Source: CAD feature listing. Evaluate the final solid. Frame: model axes, mm. A direction names the side the tool comes from. Coordinates: 2 decimals unless noted, no trailing zeros. Order: outer loops, then holes, each group sorted by start corner. A loop starts at its lowest first (then second) coordinate and runs counter-clockwise, first axis right, second up. Notation, with made-up numbers: (27, 12.25) -> (63, 12.25) arc R13 cw to (63, 16.25) -> close; hole circle Ø5 at (23.5, 1). An arc over 180 degrees is marked (long way). Write each question's results on one line, items separated by ' | '. Start each with the question number.
Solid Edge part; units mm, degrees
sketch "Sketch1" plane through (0, 0, 0) normal (0, -1, 0) x (1, 0, 0)
  line L0 (21, -100) -> (21, 100)
  line L1 (21, 100) -> (-21, 100)
  line L2 (-21, 100) -> (-21, -100)
  line L3 (-21, -100) -> (21, -100)
extrude "Protrusion1" add sketch "Sketch1" along normal blind 10
sketch "Sketch2" plane through (0, 0, 0) normal (0, -1, 0) x (1, 0, 0)
  circle A0 centre (16, -56.5) radius 2
  circle A1 centre (-16, -56.5) radius 2
  circle A2 centre (-16, -90) radius 2
  circle A3 centre (16, -90) radius 2
extrude "ExtrudedProtrusion_2" add sketch "Sketch2" against normal blind 7
sketch "Sketch3" plane through (0, -10, 0) normal (0, -1, 0) x (0, 0, -1)
  line L0 (90, 21) -> (90, -21)
  line L1 (90, -21) -> (100, -21)
  line L2 (100, -21) -> (100, 21)
  line L3 (100, 21) -> (90, 21)
extrude "ExtrudedProtrusion_3" add sketch "Sketch3" along normal blind 47
sketch "Sketch4" plane through (0, -29.5, -90) normal (0, 0, 1) x (0, 1, 0)
  circle A0 centre (-17.5, 0) radius 6
  circle A1 centre (2.5, 0) radius 4.6
extrude "Cutout1" cut sketch "Sketch4" against normal up to next
sketch "Sketch5" plane through (0, -29.5, -90) normal (0, 0, 1) x (0, 1, 0)
  circle A0 centre (2.5, 0) radius 4.6
  circle A1 centre (2.5, 0) radius 11.25
extrude "ExtrudedCutout_2" cut sketch "Sketch5" against normal blind 7.5
sketch "Sketch6" plane through (0, -28.5, -100) normal (0, 0, -1) x (0, 1, 0)
  line L0 (28.5, 21) -> (-28.5, 21)
  line L1 (-28.5, 21) -> (-28.5, -21)
  line L2 (-28.5, -21) -> (28.5, -21)
  line L3 (28.5, -21) -> (28.5, 21)
  circle A0 centre (1.5, 0) radius 4.6
  circle A1 centre (-18.5, 0) radius 6
extrude "Protrusion2" add sketch "Sketch6" along normal blind 1.7
sketch "Sketch7" plane through (0, -28.5, -100) normal (0, 0, -1) x (0, 1, 0)
  circle A0 centre (9.5, 17.5) radius 2
  circle A1 centre (9.5, -17.5) radius 2
extrude "Cutout2" cut sketch "Sketch7" along normal up to next
sketch "Sketch8" plane through (0, -28.5, -100) normal (0, 0, -1) x (0, 1, 0)
  circle A0 centre (9.5, 17.5) radius 2
  circle A1 centre (9.5, -17.5) radius 2
extrude "Cutout3" cut sketch "Sketch8" against normal up to next
sketch "Sketch9" plane through (0, -5, 100) normal (0, 0, 1) x (0, 1, 0)
  line L0 (-5, 21) -> (-5, -21)
  line L1 (-5, -21) -> (5, -21)
  line L2 (5, -21) -> (5, 21)
  line L3 (5, 21) -> (-5, 21)
extrude "ExtrudedProtrusion_6" add sketch "Sketch9" along normal blind 9
sketch "Sketch10" plane through (0, -5, 109) normal (0, 0, 1) x (0, 1, 0)
  circle A0 centre (0, 16) radius 2.25
  circle A1 centre (0, -16) radius 2.25
extrude "ExtrudedCutout_5" cut sketch "Sketch10" against normal blind 10
(1) Reachability of faces 1 (the flat face through (0, -10, 11)), 2 (the cylindrical face through (16, 3, -88)), 3 (the cylindrical face through (4.31, -16.61, -93.7)) from +Z, -Z, +X, -X, +Y, -Y: full face, straight path, thin tool, end or side. Return the list, or none.
(2) First-contact query: P1, Ø2, axis at x = -15.5, y = -4, coming from the +Z side; P2, Ø3, axis at x = 17.5, y = -19, coming from the -Z side; P3, Ø1, axis at x = 11, z = 9, coming from the +Y side; P4, Ø11, axis at x = -3.5, y = -29, coming from the +Z side. Flat tips, straight axial feed; report the tip coordinate or a pass-through.
(3) Section B-B on x = 0. Return the cut outline in (y, z).
(4) Section A-A on y = -27. Return the cut outline in (x, z).
(5) Line query: L1, parallel to Y at x = 0, z = -95.5; L2, parallel to X at y = -5, z = 104.25; L3, parallel to Y at x = 16, z = 103. Output: solid intervals per line, ascending.
(6) Section D-D on y = -47. Return the cut outline in (x, z).
(7) Section C-C on y = -36. Return the cut outline in (x, z), then the cut area to 3 significant figures.
(8) Draft query along X for faces 4 (the cylindrical face through (-16, 3, -88)), 5 (the flat face through (0, -5, 109)), 6 (the flat face through (-21, -9, -11)). Return one class per face: released by +X, released by -X, zero draft, split by the parting line, or undercut.
Results list:
1) face 1: +Z, +X, -X, -Y | face 2: +Y | face 3: +Z
2) P1: stops at z = 99 | P2: passes through | P3: stops at y = 0 | P4: stops at z = -97.5
3) outline: (-57, -101.7) -> (-53, -101.7) -> (-53, -90) -> (-57, -90) -> close; (-41, -101.7) -> (-31.6, -101.7) -> (-31.6, -97.5) -> (-38.25, -97.5) -> (-38.25, -90) -> (-41, -90) -> close; (-22.4, -101.7) -> (0, -101.7) -> (0, 109) -> (-10, 109) -> (-10, -90) -> (-15.75, -90) -> (-15.75, -97.5) -> (-22.4, -97.5) -> close
4) outline: (-21, -101.7) -> (-4.6, -101.7) -> (-4.6, -97.5) -> (-11.25, -97.5) -> (-11.25, -90) -> (-21, -90) -> close; (4.6, -101.7) -> (21, -101.7) -> (21, -90) -> (11.25, -90) -> (11.25, -97.5) -> (4.6, -97.5) -> close
5) L1: y = -57 to -53, -41 to -38.25, -15.75 to 0 | L2: x = -21 to -18.25, -13.75 to 13.75, 18.25 to 21 | L3: y = -10 to -7.25, -2.75 to 0
6) outline: (-21, -101.7) -> (-6, -101.7) -> (-6, -90) -> (-21, -90) -> close; (6, -101.7) -> (21, -101.7) -> (21, -90) -> (6, -90) -> close
7) outline: (-21, -101.7) -> (21, -101.7) -> (21, -90) -> (6.75, -90) -> (6.75, -97.5) -> (-6.75, -97.5) -> (-6.75, -90) -> (-21, -90) -> close | area: 390 mm²
8) face 4: undercut | face 5: zero draft | face 6: released by -X
